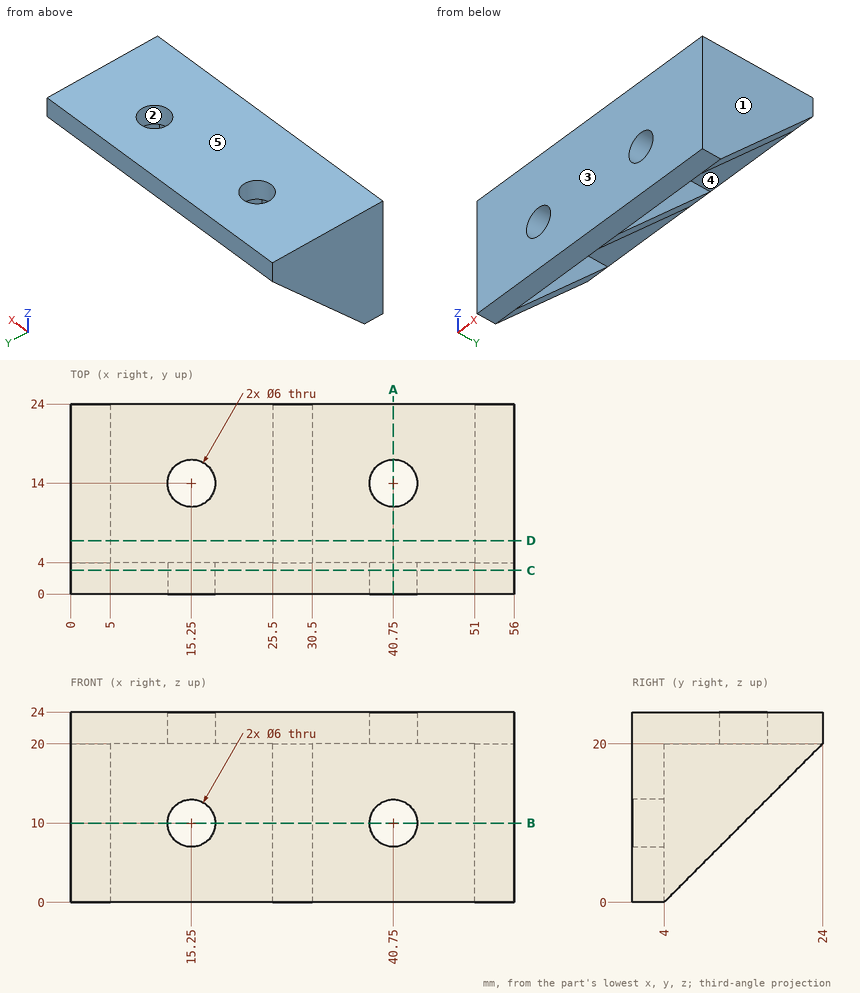
Input: dimensioned drawing with shaded views. Units: mm. Origin: part minimum x, y, z. A direction names the side the tool comes from. Coordinates: 2 decimals unless noted, no trailing zeros. Write each loop counter-clockwise with the first axis right and the second up, starting at its lowest first coordinate (ties: lowest second). Pieces come first, ordered by that corner, then holes. Notation, with made-up numbers: (15, 75.25) -> (54, 75.25) arc R9 cw to (54, 90.25) -> close; hole circle Ø4 at (68.5, -5.75). An arc over 180 degrees is marked (long way). Return JSON: item names as keys, results as strings. Group by question number.
1) Set-up query: the marked faces 4 and 5. Return all of +Z, -Z, +X, -X, +Y, -Y with unobstructed straight access to the full face (end or side cutting, diameter ignored); none if empty.
2) Mould query, pull axis X, two halves, no side actions, for the marked faces 1, 2 and 3. Classes: +X half, -X half, draft (parallel to the pull), parting line (faces both ways), or undercut.
3) Section query A-A, the plane x = 40.75. Return loops of the section in (y, z).
4) Section query D-D, the plane y = 6.75. Return loops of the section in (x, z), plus the area to 3 significant figures.
5) Section query B-B, the plane z = 10. Return loops of the section in (x, y).
6) Ray query, line 1 along X through (y, z) = (5.5, 15); line 2 along Z through (x, y) = (15.25, 1.25); line 3 along Y through (x, z) = (15.25, 21.05). Return the intervals inside material, ascending.
7) Section query C-C, the plane y = 3. Return loops of the section in (x, z).
8) Contact query for flat-ended pins moving along their axis: P1, Ø6, axis at x = 14.5, z = 14.5, coming from the +Y side; P2, Ø9.5, axis at x = 15.25, y = 14, coming from the -Z side. Output: stop coordinate, or through.
From the geometry:
{
 "1": {"face 4": "-Z, +Y", "face 5": "+Z, +X, -X, +Y, -Y"},
 "2": {"face 1": "+X half", "face 2": "undercut", "face 3": "draft"},
 "3": {"outline": "(0, 0) -> (4, 0) -> (4, 7) -> (0, 7) -> close; (0, 13) -> (4, 13) -> (4, 20) -> (11, 20) -> (11, 24) -> (0, 24) -> close; (17, 20) -> (24, 20) -> (24, 24) -> (17, 24) -> close"},
 "4": {"outline": "(0, 2.75) -> (5, 2.75) -> (5, 20) -> (25.5, 20) -> (25.5, 2.75) -> (30.5, 2.75) -> (30.5, 20) -> (51, 20) -> (51, 2.75) -> (56, 2.75) -> (56, 24) -> (0, 24) -> close", "area": "483 mm²"},
 "5": {"outline": "(0, 0) -> (12.25, 0) -> (12.25, 4) -> (5, 4) -> (5, 14) -> (0, 14) -> close; (18.25, 0) -> (37.75, 0) -> (37.75, 4) -> (30.5, 4) -> (30.5, 14) -> (25.5, 14) -> (25.5, 4) -> (18.25, 4) -> close; (43.75, 0) -> (56, 0) -> (56, 14) -> (51, 14) -> (51, 4) -> (43.75, 4) -> close"},
 "6": {"line 1": "0 to 5, 25.5 to 30.5, 51 to 56", "line 2": "0 to 7, 13 to 24", "line 3": "0 to 11, 17 to 24"},
 "7": {"outline": "(0, 0) -> (56, 0) -> (56, 24) -> (0, 24) -> close; hole circle Ø6 at (15.25, 10); hole circle Ø6 at (40.75, 10)"},
 "8": {"P1": "y = 4", "P2": "z = 20"}
}
